from build123d import *

# Parameters (mm, degrees)
ESQUISSE1_W             = 60
ESQUISSE1_H             = 50
BOSS_EXTRU_1_DEPTH      = 5
ESQUISSE2_R             = 2
BOSS_EXTRU_2_DEPTH      = 40
ESQUISSE3_R             = 2
ENL_V_MAT_EXTRU_1_DEPTH = 88.749643874
CONG_1_R                = 2
CONG_2_R                = 2
ENL_V_START             = -1.5
ESQUISSE4_R             = 3.75
ESQUISSE4_R_2           = 2
ENL_V_MAT_EXTRU_5_DEPTH = 1.5
CONG_5_R                = 2
CONG_6_R                = 2
CONG_7_R                = 2
CONG_8_R                = 2


with BuildPart() as part:
    # Esquisse1 → Boss.-Extru.1 (new, symmetric)
    with BuildSketch(Plane.XY):
        with Locations((30, -25)):
            Rectangle(ESQUISSE1_W, ESQUISSE1_H)
    extrude(amount=BOSS_EXTRU_1_DEPTH, both=True)

    # Esquisse2 → Boss.-Extru.2 (add)
    with BuildSketch(Plane.XY.offset(5)):
        with Locations((5, -12.5)):
            Circle(ESQUISSE2_R)
        with Locations(Location((5, -37.5, 0), (0, 0, 180))):
            Circle(ESQUISSE2_R)
        with Locations((55, -37.5)):
            Circle(ESQUISSE2_R)
        with Locations(Location((55, -12.5, 0), (0, 0, 180))):
            Circle(ESQUISSE2_R)
    extrude(amount=BOSS_EXTRU_2_DEPTH)

    # Esquisse3 → Enlèv. mat.-Extru.1 (cut, through all)
    with BuildSketch(Plane.XY.offset(5)):
        with Locations((30, -25)):
            Circle(ESQUISSE3_R)
    extrude(amount=-ENL_V_MAT_EXTRU_1_DEPTH, mode=Mode.SUBTRACT)

    # Congé1
    cong_1_edges = [part.edges().sort_by_distance(p)[0] for p in [
        (0, 0, 0),
    ]]
    fillet(cong_1_edges, radius=CONG_1_R)

    # Congé2
    cong_2_edges = [part.edges().sort_by_distance(p)[0] for p in [
        (60, 0, 0),
        (60, -50, 0),
        (0, -50, 0),
    ]]
    fillet(cong_2_edges, radius=CONG_2_R)

    # Esquisse4 → Enlèv. mat.-Extru.5 (cut)
    # profile 1 of 4: a face of its own
    with BuildSketch(Plane.XY.offset(5).offset(ENL_V_START)):
        with Locations((5, -37.5)):
            Circle(ESQUISSE4_R)
        with Locations(Location((5, -37.5, 0), (0, 0, 180))):
            Circle(ESQUISSE4_R_2, mode=Mode.SUBTRACT)
    # profile 2 of 4: a face of its own
    with BuildSketch(Plane.XY.offset(5).offset(ENL_V_START)):
        with Locations(Location((5, -12.5, 0), (0, 0, 180))):
            Circle(ESQUISSE4_R)
        with Locations((5, -12.5)):
            Circle(ESQUISSE4_R_2, mode=Mode.SUBTRACT)
    # profile 3 of 4: a face of its own
    with BuildSketch(Plane.XY.offset(5).offset(ENL_V_START)):
        with Locations((55, -12.5)):
            Circle(ESQUISSE4_R)
        with Locations(Location((55, -12.5, 0), (0, 0, 180))):
            Circle(ESQUISSE4_R_2, mode=Mode.SUBTRACT)
    # profile 4 of 4: a face of its own
    with BuildSketch(Plane.XY.offset(5).offset(ENL_V_START)):
        with Locations(Location((55, -37.5, 0), (0, 0, 180))):
            Circle(ESQUISSE4_R)
        with Locations((55, -37.5)):
            Circle(ESQUISSE4_R_2, mode=Mode.SUBTRACT)
    extrude(amount=ENL_V_MAT_EXTRU_5_DEPTH, mode=Mode.SUBTRACT)

    # Congé5
    # the kernel refuses this fillet: 2 mm, written as the material it adds along each edge
    with BuildSketch(Plane(origin=(55, -37.5, 3.5), x_dir=(1, 0, 0), z_dir=(0, -1, 0))) as cong_5_piece_1:
        with BuildLine():
            CenterArc((4, 1.984313483), CONG_5_R, 180, 82.819244219)
            Line((2, 1.984313483), (1.96, 1.984313483))
            Line((1.96, 1.984313483), (1.96, 0))
            Line((1.96, 0), (2, -0.04))
            ThreePointArc((2, -0.04), (2.875, -0.04), (3.745, -0.03968627))
            Line((3.745, -0.03968627), (3.75, 0))
        make_face()
    revolve(axis=Axis((55, -37.5, 3.5), (0, 0, 1)))

    # Congé6
    # the kernel refuses this fillet: 2 mm, written as the material it adds along each edge
    with BuildSketch(Plane(origin=(55, -12.5, 3.5), x_dir=(-1, 0, 0), z_dir=(0, 1, 0))) as cong_6_piece_1:
        with BuildLine():
            CenterArc((4, 1.984313483), CONG_6_R, 180, 82.819244219)
            Line((2, 1.984313483), (1.96, 1.984313483))
            Line((1.96, 1.984313483), (1.96, 0))
            Line((1.96, 0), (2, -0.04))
            ThreePointArc((2, -0.04), (2.875, -0.04), (3.745, -0.03968627))
            Line((3.745, -0.03968627), (3.75, 0))
        make_face()
    revolve(axis=Axis((55, -12.5, 3.5), (0, 0, 1)))

    # Congé7
    # the kernel refuses this fillet: 2 mm, written as the material it adds along each edge
    with BuildSketch(Plane(origin=(5, -12.5, 3.5), x_dir=(1, 0, 0), z_dir=(0, -1, 0))) as cong_7_piece_1:
        with BuildLine():
            CenterArc((4, 1.984313483), CONG_7_R, 180, 82.819244219)
            Line((2, 1.984313483), (1.96, 1.984313483))
            Line((1.96, 1.984313483), (1.96, 0))
            Line((1.96, 0), (2, -0.04))
            ThreePointArc((2, -0.04), (2.875, -0.04), (3.745, -0.03968627))
            Line((3.745, -0.03968627), (3.75, 0))
        make_face()
    revolve(axis=Axis((5, -12.5, 3.5), (0, 0, 1)))

    # Congé8
    # the kernel refuses this fillet: 2 mm, written as the material it adds along each edge
    with BuildSketch(Plane(origin=(5, -37.5, 3.5), x_dir=(-1, 0, 0), z_dir=(0, 1, 0))) as cong_8_piece_1:
        with BuildLine():
            CenterArc((4, 1.984313483), CONG_8_R, 180, 82.819244219)
            Line((2, 1.984313483), (1.96, 1.984313483))
            Line((1.96, 1.984313483), (1.96, 0))
            Line((1.96, 0), (2, -0.04))
            ThreePointArc((2, -0.04), (2.875, -0.04), (3.745, -0.03968627))
            Line((3.745, -0.03968627), (3.75, 0))
        make_face()
    revolve(axis=Axis((5, -37.5, 3.5), (0, 0, 1)))


solid = part.part
For this review, take the finished solid that the model builds, in its own axes (mm). A direction names the side the tool comes from. Round coordinates to 2 decimals unless told otherwise and drop trailing zeros. Order: outer loops, then holes, each group sorted by start corner. A loop starts at its lowest first (then second) coordinate and runs counter-clockwise, first axis right, second up. Notation, with made-up numbers: (-35, -11.75) -> (17, -11.75) arc R24 cw to (17, 19.25) -> close; hole circle Ø6 at (-23.5, 56.25). An arc over 180 degrees is marked (long way). Write item = value, one per line. Start each with the question number.
1) Take a section at C-C on z = 22.5. State the section outline as (x, y) points, plus the area to 3 significant figures.
2) Take a section at D-D on x = 55. State the section outline as (y, z) points.
3) To check wall thickness, follow line 1 (Y direction, x = 30, z = 1); line 2 (X direction, y = -12.5, z = 4.45); line 3 (Y direction, x = 5, z = 4). State the ranges of each line that lie inside material, in increasing order. Write a range as from..to.
4) Take a section at A-A on x = 30. State the section outline as (y, z) points.
5) Tool access review of faces 1 (the face through (30, -19, -5)), 2 (the face through (3.526, -11.148, 24.966)): name each direction out of +Z, -Z, +X, -X, +Y, -Y from which nothing blocks a thin tool from reaching the whole face with its end or side.
6) Insertion check: pin 1 (12 mm diameter, centred on y = -43, z = 26, fed in from +X); pin 2 (2 mm diameter, centred on x = 31.5, y = -40.5, fed in from +Z); pin 3 (25 mm diameter, centred on x = 15.5, y = -14.5, fed in from +Z). Each pin has a flat end and moves straight along its axis. Give the tip position at first contact, or say it passes through.
7) Take a section at B-B on y = -25. State the section outline as (x, z) points, plus the area to 3 significant figures.
Verdict:
q1.outline = circle Ø4 at (5, -37.5); circle Ø4 at (5, -12.5); circle Ø4 at (55, -37.5); circle Ø4 at (55, -12.5)
q1.area = 50.3 mm2
q2.outline = (-50, -5) -> (0, -5) -> (0, 5) -> (-8.75, 5) -> (-8.75, 3.5) arc R2 cw to (-10.5, 5.48) -> (-10.5, 45) -> (-14.5, 45) -> (-14.5, 5.48) arc R2 cw to (-16.25, 3.5) -> (-16.25, 5) -> (-33.75, 5) -> (-33.75, 3.5) arc R2 cw to (-35.5, 5.48) -> (-35.5, 45) -> (-39.5, 45) -> (-39.5, 5.48) arc R2 cw to (-41.25, 3.5) -> (-41.25, 5) -> (-50, 5) -> close
q3.line_1 = -50..-27, -23..0
q3.line_2 = 0..1.25, 2.71..7.29, 8.75..51.25, 52.71..57.29, 58.75..60
q3.line_3 = -50..-41.25, -40.16..-34.84, -33.75..-16.25, -15.16..-9.84, -8.75..0
q4.outline = (-50, -5) -> (-27, -5) -> (-27, 5) -> (-50, 5) -> close; (-23, -5) -> (0, -5) -> (0, 5) -> (-23, 5) -> close
q5.face_1 = -Z, +X, -X, +Y, -Y
q5.face_2 = +Z
q6.pin_1 = 57
q6.pin_2 = 5
q6.pin_3 = 45
q7.outline = (0, -5) -> (28, -5) -> (28, 5) -> (0, 5) -> close; (32, -5) -> (60, -5) -> (60, 5) -> (32, 5) -> close
q7.area = 560 mm2
